Build history of the part. All positions in model axes, mm. Round coordinates to 2 decimals unless told otherwise and drop trailing zeros. Order: outer loops, then holes, each group sorted by start corner. A loop starts at its lowest first (then second) coordinate and runs counter-clockwise, first axis right, second up. Notation, with made-up numbers: (17, -37.5) -> (26, -37.5) arc R18 cw to (26, -13.5) -> close; hole circle Ø7 at (-19, -15). An arc over 180 degrees is marked (long way). Answer as CSV lines item,"result". Start each with the question number.
```python
from build123d import *

# Parameters (mm, degrees)
SKETCH_1_W          = 15
SKETCH_1_H          = 30
EXTRUDE_1_DEPTH     = 15
SKETCH_2_R          = 5.35
CUT_EXTRUDE_1_DEPTH = 15
SKETCH_4_R          = 5.35
CUT_EXTRUDE_2_DEPTH = 15
SKETCH_5_R          = 1.5
CUT_EXTRUDE_3_DEPTH = 20
SKETCH_7_R          = 1.5
CUT_EXTRUDE_4_DEPTH = 20
SKETCH_8_R          = 1.5
CUT_EXTRUDE_5_DEPTH = 50


with BuildPart() as part:
    # 草图1 → 凸台-拉伸1 (new body)
    with BuildSketch(Plane(origin=(0, 0, 0), x_dir=(0, 0, -1), z_dir=(1, 0, 0))):
        Rectangle(SKETCH_1_W, SKETCH_1_H)
    extrude(amount=EXTRUDE_1_DEPTH)

    # 草图2 → 切除-拉伸1 (cut)
    with BuildSketch(Plane(origin=(15, 0, 0), x_dir=(0, 0, -1), z_dir=(1, 0, 0))):
        with Locations((0, -7.537865607)):
            Circle(SKETCH_2_R)
    extrude(amount=-CUT_EXTRUDE_1_DEPTH, mode=Mode.SUBTRACT)

    # 草图4 → 切除-拉伸2 (cut)
    with BuildSketch(Plane.XY.offset(7.5)):
        with Locations((7.5, 8.242569868)):
            Circle(SKETCH_4_R)
    extrude(amount=-CUT_EXTRUDE_2_DEPTH, mode=Mode.SUBTRACT)

    # 草图5 → 切除-拉伸3 (cut)
    with BuildSketch(Plane.XY.offset(7.5)):
        with Locations((7.314343795, -7.54)):
            Circle(SKETCH_5_R)
    extrude(amount=-CUT_EXTRUDE_3_DEPTH, mode=Mode.SUBTRACT)

    # 草图7 → 切除-拉伸4 (cut)
    with BuildSketch(Plane(origin=(15, 0, 0), x_dir=(0, 0, -1), z_dir=(1, 0, 0))):
        with Locations((0, 8.24)):
            Circle(SKETCH_7_R)
    extrude(amount=-CUT_EXTRUDE_4_DEPTH, mode=Mode.SUBTRACT)

    # 草图8 → 切除-拉伸5 (cut)
    with BuildSketch(Plane.XZ.offset(15)):
        with Locations(Location((7.5, 0, 0), (0, 0, 270))):
            Circle(SKETCH_8_R)
    extrude(amount=-CUT_EXTRUDE_5_DEPTH, mode=Mode.SUBTRACT)


solid = part.part
```
Q1. Slice it at A-A, the plane x = 2.75. Write the cut outline in (y, z), plus the area to 3 significant figures.
Q2. Slice it at C-C, the plane y = 13. Write the cut outline in (x, z), plus the area to 3 significant figures.
Q3. Two-plate mould, pull along Z, no slides. Class faces 1 (the face through (8.745, -7.089, -6.301)), 2 (the face through (6, 0, 0)), 3 (the face through (7, -4, -7.5)): +Z half, -Z half, draft (parallel to the pull), parting line (faces both ways), or undercut.
Q4. Slice it at D-D, the plane z = 0.5. Write the cut outline in (x, y), plus the area to 3 significant figures.
Q5. Probe L1, parallel to Z at x = 13.6, y = 8.24; L2, parallel to Y at x = 8.5, z = -2; L3, parallel to X at y = 13.8, z = 0. List the from-to ranges inside material, lowest first.
Q6. Slice it at B-B, the plane z = 2.25. Write the cut outline in (x, y).
Solutions:
1,outline,"(-15, -7.5) -> (5.78, -7.5) -> (5.78, 7.5) -> (-15, 7.5) -> close; (10.7, -7.5) -> (15, -7.5) -> (15, 7.5) -> (10.7, 7.5) -> close; hole circle Ø10.7 at (-7.54, 0)"
1,area,"286 mm2"
2,outline,"(0, -7.5) -> (5.05, -7.5) -> (5.05, 7.5) -> (0, 7.5) -> close; (9.95, -7.5) -> (15, -7.5) -> (15, 7.5) -> (9.95, 7.5) -> close"
2,area,"152 mm2"
3,face 1,"draft"
3,face 2,"undercut"
3,face 3,"-Z half"
4,outline,"(0, -15) -> (6.09, -15) -> (6.09, -12.86) -> (0, -12.86) -> close; (0, -2.21) -> (6.09, -2.21) -> (6.09, 3.08) arc R5.35 cw to (2.34, 6.83) -> (0, 6.83) -> close; (0, 9.65) -> (2.34, 9.65) arc R5.35 cw to (6.09, 13.4) -> (6.09, 15) -> (0, 15) -> close; (8.91, -15) -> (15, -15) -> (15, -12.86) -> (8.91, -12.86) -> close; (8.91, -2.21) -> (15, -2.21) -> (15, 6.83) -> (12.66, 6.83) arc R5.35 cw to (8.91, 3.08) -> close; (8.91, 13.4) arc R5.35 cw to (12.66, 9.65) -> (15, 9.65) -> (15, 15) -> (8.91, 15) -> close"
4,area,"163 mm2"
5,L1,"z = -7.5 to -1.5, 1.5 to 7.5"
5,L2,"y = -15 to -12.5, -2.58 to 2.99, 13.5 to 15"
5,L3,"x = 0 to 6, 9 to 15"
6,outline,"(0, -15) -> (15, -15) -> (15, -12.39) -> (0, -12.39) -> close; (0, -2.68) -> (15, -2.68) -> (15, 15) -> (0, 15) -> close; hole circle Ø10.7 at (7.5, 8.24)"
